from build123d import *

# Parameters (mm, degrees)
CROQUIS3_R              = 12
CROQUIS3_R_2            = 3.25
SALIENTE_EXTRUIR1_DEPTH = 1
MATRIZL1_COUNT          = 8
MATRIZL1_PITCH          = 3
CROQUIS5_R              = 1.55
CORTAR_EXTRUIR1_DEPTH   = 2
MATRIZC1_COUNT          = 6
CHAFL_N3_SIZE           = 0.3
CHAFL_N3_SIZE2          = 0.519615242
CROQUIS6_R              = 7.15
CORTAR_EXTRUIR2_DEPTH   = 1
CHAFL_N2_SIZE           = 0.15
CHAFL_N2_SIZE2          = 0.259807621
CHAFL_N4_SIZE           = 1
CHAFL_N4_SIZE2          = 1.732050808


with BuildPart() as part:
    # Croquis1 → Revolución1 (revolve)
    with BuildSketch(Plane.XY):
        Polygon((0, 0), (6, 0), (6, 9), (5.25, 9), (5.25, 12), (4.75, 12), (4.75, 22), (8, 22), (8, 35), (12.5, 35), (12.5, 37), (0, 37), align=None)
    revolve(axis=Axis((0, 37, 0), (0, -1, 0)))

    # Croquis2 → Cortar-Revolución1 (revolve, cut)
    with BuildSketch(Plane.XY):
        Polygon((0, 0), (2.5, 0), (2.5, 12), (1.7, 12), (1.7, 14), (3.25, 14), (3.25, 29.5), (5.25, 29.5), (5.25, 32), (6.75, 32), (6.75, 37), (0, 37), align=None)
    revolve(axis=Axis((0, 0, 0), (0, 1, 0)), mode=Mode.SUBTRACT)

    # Croquis3 → Saliente-Extruir1 (add)
    with BuildSketch(Plane.XZ):
        Circle(CROQUIS3_R)
        Circle(CROQUIS3_R_2, mode=Mode.SUBTRACT)
    saliente_extruir1 = extrude(amount=-SALIENTE_EXTRUIR1_DEPTH)

    # MatrizL1: Saliente-Extruir1 ×8
    with Locations(*[(0, i * MATRIZL1_PITCH, 0) for i in range(1, MATRIZL1_COUNT)]):
        add(saliente_extruir1)

    # Croquis5 → Cortar-Extruir1 (cut)
    with BuildSketch(Plane(origin=(0, 37, 0), x_dir=(1, 0, 0), z_dir=(0, 1, 0))):
        with Locations((0, 10.125)):
            Circle(CROQUIS5_R)
    cortar_extruir1 = extrude(amount=-CORTAR_EXTRUIR1_DEPTH, mode=Mode.SUBTRACT)

    # MatrizC1: Cortar-Extruir1 ×6 about axis
    matrizc1_axis = Axis((0, 0, 0), (0, 1, 0))
    for i in range(1, MATRIZC1_COUNT):
        add(cortar_extruir1.rotate(matrizc1_axis, i * 360 / MATRIZC1_COUNT), mode=Mode.SUBTRACT)

    # Chaflán3
    chafl_n3_edges = [part.edges().sort_by_distance(p)[0] for p in [
        (-1.7, 14, 0),
    ]]
    chafl_n3_side = [part.faces().sort_by_distance(p)[0] for p in [
        (-1.791923882, 14, 0),
    ]]
    chamfer(chafl_n3_edges, length=CHAFL_N3_SIZE, length2=CHAFL_N3_SIZE2, reference=chafl_n3_side[0])

    # Croquis6 → Cortar-Extruir2 (cut)
    with BuildSketch(Plane(origin=(0, 37, 0), x_dir=(1, 0, 0), z_dir=(0, 1, 0))):
        Circle(CROQUIS6_R)
    extrude(amount=-CORTAR_EXTRUIR2_DEPTH, mode=Mode.SUBTRACT)

    # Chaflán2
    chafl_n2_edges = [part.edges().sort_by_distance(p)[0] for p in [
        (-1.7, 12, 0),
    ]]
    chafl_n2_side = [part.faces().sort_by_distance(p)[0] for p in [
        (-2.429289322, 12, 0),
    ]]
    chamfer(chafl_n2_edges, length=CHAFL_N2_SIZE, length2=CHAFL_N2_SIZE2, reference=chafl_n2_side[0])

    # Chaflán4
    chafl_n4_edges = [part.edges().sort_by_distance(p)[0] for p in [
        (-3.25, 29.5, 0),
    ]]
    chafl_n4_side = [part.faces().sort_by_distance(p)[0] for p in [
        (-3.398492424, 29.5, 0),
    ]]
    chamfer(chafl_n4_edges, length=CHAFL_N4_SIZE, length2=CHAFL_N4_SIZE2, reference=chafl_n4_side[0])


solid = part.part
Work out the finished part from the listing and answer in its coordinate system (mm). A direction names the side the tool comes from. Round coordinates to 2 decimals unless told otherwise and drop trailing zeros. Order: outer loops, then holes, each group sorted by start corner. A loop starts at its lowest first (then second) coordinate and runs counter-clockwise, first axis right, second up. Notation, with made-up numbers: M 13.25,20.5 L 37.25,20.5 A19 ccw 37.25,24.5 Z; hole C -17.75,72.25 d3. An arc over 180 degrees is marked long. Put each result on its own line as item: value. Start each with the question number.
Q1. For a pull along Y with two mould halves and no side action, classify faces 1 (the flat face through (5, 16, 0)), 2 (the flat face through (-2, 29.5, 4)), 3 (the cylindrical face through (-0.336, 36.014, -8.612)) as pulls with the +Y half, pulls with the -Y half, needs draft (parallel to the pull), parting line crosses it, or undercut.
Q2. Straight lines are drawn through the part: L1, parallel to Y at x = 5.5, z = -1; L2, parallel to Z at x = 0, y = 20; L3, parallel to Z at x = 0, y = 30.6. For each, find the intervals that lie inside material, in ascending order. Write a range as [from, to].
Q3. Section C-C, the plane y = 24 is taken. Write down the section's boundary in (x, z).
Q4. Section B-B, the plane y = 5 is taken. Write down the section's boundary in (x, z), and give its area (3 significant figures).
Q5. A tool of negligible diameter and unlimited length cuts with its end or side. For faces 4 (the cylindrical face through (-11.99, 6.49, 0.53)), 5 (the flat face through (5, 15, 0)), 6 (the cylindrical face through (11.923, 36.014, 3.755)), 7 (the flat face through (0, 0, 3)), 8 (the cylindrical face through (10.247, 36.014, 4.597)), from which of +Z, -Z, +X, -X, +Y, -Y can it reach the whole face along a straight path? Write none if from no direction.
Q6. Flat-ended cylindrical pins translate along their axes: pin 1 (5 mm diameter, centred on x = 4, y = 22, fed in from -Z); pin 2 (13 mm diameter, centred on x = 0, z = 0, fed in from -Y); pin 3 (3 mm diameter, centred on y = 26, z = 5.5, fed in from -X); pin 4 (5 mm diameter, centred on x = 0, z = 0, fed in from +Y). Find the tip coordinate at first contact, or state that the pin passes through.
Q7. Section A-A, the plane x = 0 is taken. Give the number of separate pieces and of enclosed holes in the cut face, and give its area (3 significant figures).
Findings below:
1. face 1: undercut
1. face 2: pulls with the +Y half
1. face 3: needs draft
2. L1: y = [0, 10], [12, 13], [15, 16], [18, 19], [21, 32]
2. L2: z = [-4.75, -3.25], [3.25, 4.75]
2. L3: z = [-8, -5.25], [5.25, 8]
3. outline: C 0,0 d16; hole C 0,0 d6.5
4. outline: C 0,0 d12; hole C 0,0 d5
4. area: 93.5 mm^2
5. face 4: -Y
5. face 5: none
5. face 6: +Y, -Y
5. face 7: +Z, -Z, +X, -X, -Y
5. face 8: +Y
6. pin 1: stops at z = -11.91
6. pin 2: stops at y = 0
6. pin 3: stops at x = -6.93
6. pin 4: stops at y = 14
7. separate pieces: 4
7. enclosed holes: 0
7. area: 324 mm^2
